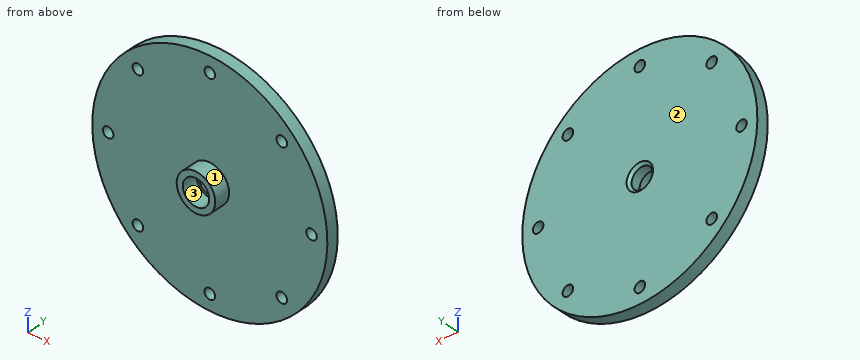
```python
from build123d import *

# Parameters (mm, degrees)
SKETCH_1_R          = 22.25
SKETCH_1_R_2        = 2
EXTRUDE_1_DEPTH     = 2.25
SKETCH_3_R          = 3.65
SKETCH_3_R_2        = 2.5
EXTRUDE_2_DEPTH     = 3
CHAMFER_1_SIZE      = 0.5
SKETCH_4_R          = 1
CUT_EXTRUDE_3_DEPTH = 32.90121471


with BuildPart() as part:
    # Эскиз1 → Вытянуть1 (new body)
    with BuildSketch(Plane(origin=(0, 0, 0), x_dir=(1, 0, 0), z_dir=(0, 1, 0))):
        with Locations(Location((0, 0, 0), (0, 0, 270))):
            Circle(SKETCH_1_R)
        with Locations(Location((0, 0, 0), (0, 0, 270))):
            Circle(SKETCH_1_R_2, mode=Mode.SUBTRACT)
    extrude(amount=EXTRUDE_1_DEPTH)

    # Эскиз3 → Вытянуть2 (add)
    with BuildSketch(Plane.XZ):
        with Locations(Location((0, 0, 0), (0, 0, 90))):
            Circle(SKETCH_3_R)
        with Locations(Location((0, 0, 0), (0, 0, 270))):
            Circle(SKETCH_3_R_2, mode=Mode.SUBTRACT)
    extrude(amount=EXTRUDE_2_DEPTH)

    # Фаска1
    chamfer_1_edges = [part.edges().sort_by_distance(p)[0] for p in [
        (0, 2.25, -2),
    ]]
    chamfer(chamfer_1_edges, length=CHAMFER_1_SIZE)

    # Эскиз4 → Вытянуть3 (cut, through all)
    with BuildSketch(Plane(origin=(0, 2.25, 0), x_dir=(1, 0, 0), z_dir=(0, 1, 0))):
        with Locations(Location((0, 19.25, 0), (0, 0, 270))):
            Circle(SKETCH_4_R)
        with Locations(Location((13.611805538, 13.611805538, 0), (0, 0, 270))):
            Circle(SKETCH_4_R)
        with Locations(Location((19.25, 0, 0), (0, 0, 270))):
            Circle(SKETCH_4_R)
        with Locations(Location((13.611805538, -13.611805538, 0), (0, 0, 270))):
            Circle(SKETCH_4_R)
        with Locations(Location((0, -19.25, 0), (0, 0, 270))):
            Circle(SKETCH_4_R)
        with Locations(Location((-13.611805538, -13.611805538, 0), (0, 0, 270))):
            Circle(SKETCH_4_R)
        with Locations(Location((-19.25, 0, 0), (0, 0, 270))):
            Circle(SKETCH_4_R)
        with Locations(Location((-13.611805538, 13.611805538, 0), (0, 0, 270))):
            Circle(SKETCH_4_R)
    extrude(amount=-CUT_EXTRUDE_3_DEPTH, mode=Mode.SUBTRACT)


solid = part.part
```
Could you check a few things on this model? Use its own coordinates, in mm. Face numbers are marked on the shaded views. Coordinates: 2 decimals unless noted, no trailing zeros. Loops run counter-clockwise (first coordinate to the right, second up) from the corner with the lowest first, then second, coordinate; pieces in that order, holes last. Notation, with made-up numbers: M 23.25,21 L 53.25,21 A31 ccw 53.25,48 Z; hole C 7.25,33 d8. An arc over 180 degrees is marked long. Put each result on its own line as item: value. Start each with the question number.
(1) I need wall thicknesses on line 1 (X direction, y = -1.8, z = 0); line 2 (Y direction, x = -1.5, z = 11); line 3 (Z direction, x = -0.5, y = 0.35). Which ranges of each line are inside material? Lowest first, please. Write a range as from..to.
(2) Suppose I cut it at B-B on x = 0. Please give me the cut outline in (y, z).
(3) Thinking about a two-plate mould opening in X: for the marked faces 1, 2 and 3, which applies, pulls with the +X half, pulls with the -X half, needs draft (parallel to the pull), parting line crosses it, or undercut?
(4) Suppose I cut it at A-A on z = 0. Please give me the cut outline in (x, y).
(5) Suppose I cut it at C-C on z = -19. Please give me the cut outline in (x, y).
(6) Suppose I cut it at D-D on y = -1.8. Please give me the cut outline in (x, z).
(7) Will this pin go through, and if not, where does the flat tip stop? P1, Ø10, axis at x = 14, z = -4, coming from the -Y side.
Solutions:
1. line 1: x = -3.65..-2.5, 2.5..3.65
1. line 2: y = 0..2.25
1. line 3: z = -22.24..-20.12, -18.38..-1.94, 1.94..18.38, 20.12..22.24
2. outline: M -3,-3.65 L 0,-3.65 L 0,-18.25 L 2.25,-18.25 L 2.25,-2.5 L 1.75,-2 L 0,-2 L 0,-2.5 L -3,-2.5 Z; M -3,2.5 L 0,2.5 L 0,2 L 1.75,2 L 2.25,2.5 L 2.25,18.25 L 0,18.25 L 0,3.65 L -3,3.65 Z; M 0,-22.25 L 2.25,-22.25 L 2.25,-20.25 L 0,-20.25 Z; M 0,20.25 L 2.25,20.25 L 2.25,22.25 L 0,22.25 Z
3. face 1: parting line crosses it
3. face 2: needs draft
3. face 3: undercut
4. outline: M -22.25,0 L -20.25,0 L -20.25,2.25 L -22.25,2.25 Z; M -18.25,0 L -3.65,0 L -3.65,-3 L -2.5,-3 L -2.5,0 L -2,0 L -2,1.75 L -2.5,2.25 L -18.25,2.25 Z; M 2,0 L 2.5,0 L 2.5,-3 L 3.65,-3 L 3.65,0 L 18.25,0 L 18.25,2.25 L 2.5,2.25 L 2,1.75 Z; M 20.25,0 L 22.25,0 L 22.25,2.25 L 20.25,2.25 Z
5. outline: M -11.58,0 L -0.97,0 L -0.97,2.25 L -11.58,2.25 Z; M 0.97,0 L 11.58,0 L 11.58,2.25 L 0.97,2.25 Z
6. outline: C 0,0 d7.3; hole C 0,0 d5
7. P1: stops at y = 0
